Check sheet for the modelled part. Datum: model origin and axes. Units: mm. A direction names the side the tool comes from. Round coordinates to 2 decimals unless told otherwise and drop trailing zeros. Write each loop counter-clockwise with the first axis right and the second up, starting at its lowest first coordinate (ties: lowest second). Pieces come first, ordered by that corner, then holes. Notation, with made-up numbers: (37, -3) - (44, -3) arc R18 ccw to (44, 2) - close; hole circle Ø11 at (75, 64.5). An arc over 180 degrees is marked (long way). Answer as a JSON object with one key per item and string values. Group by question number.
Item 1: Sectioned sample at C-C on z = 1.5. Record the boundary of the cut face in (x, y), plus the area to 3 significant figures.
Item 2: Sectioned sample at B-B on x = 0. Record the boundary of the cut face in (y, z) (3 decimals), plus the area to 3 significant figures.
Item 3: Thickness scan on line 1 (Z direction, x = 0, y = 7.2); line 2 (X direction, y = 1.25, z = 1.25). Record the ranges inside material, lowest first.
Item 4: Sectioned sample at A-A on y = 4. Record the boundary of the cut face in (x, z).
Item 5: Release check for a two-part mould opening along X. For faces 3 (the flat face through (0, 3, -1)), 4 (the flat face through (0, 0, 0)) record: pulls with the +X half, pulls with the -X half, needs draft (parallel to the pull), parting line crosses it, or undercut.
Item 6: Gauge pin test, flat ends, axial feed: P1, Ø0.5, axis at x = -0.5, z = -1.5, coming from the -Y side; P2, Ø4, axis at x = 0, z = 0, coming from the -Y side; P3, Ø1.4, axis at x = -0.5, z = -0.5, coming from the +Y side; P4, Ø1, axis at x = -1, y = 4, coming from the +Z side. Record the tip position at first contact, or that the pin passes through.
Item 7: Set-up check for faces 1 (the flat face through (0, 1, -0.45)), 2 (the cylindrical face through (1.29, 6.595, -2.024)): record each of +Z, -Z, +X, -X, +Y, -Y from which the full face is reachable in a straight line by a thin tool's end or side.
Item 8: Sectioned sample at D-D on x = 2.25. Record the boundary of the cut face in (y, z).
Autodesk Inventor part; units mm, degrees
ref_plane "YZ Plane" through (0, 0, 0) normal (1, 0, 0) x (0, 1, 0)
ref_plane "XZ Plane" through (0, 0, 0) normal (0, 1, 0) x (-1, 0, 0)
ref_plane "XY Plane" through (0, 0, 0) normal (0, 0, 1) x (1, 0, 0)
sketch "Sketch1" plane through (0, 0, 0) normal (0, 1, 0) x (-1, 0, 0)
  circle A0 centre (0, 0) radius 1.975
  circle A1 centre (0, 0) radius 3.5
  line L0 (-2.286, -0.45) -> (2.286, -0.45)
  line L1 (2.286, -0.45) -> (2.286, 0.45)
  line L2 (2.286, 0.45) -> (-2.286, 0.45)
  line L3 (-2.286, 0.45) -> (-2.286, -0.45)
  line L4 (-2.286, -0.45) -> (2.286, 0.45) construction
  line L5 (2.286, -0.45) -> (-2.286, 0.45) construction
  point P0 (-1.9231, 0.45)
  point P1 (1.9231, 0.45)
  point P2 (1.9231, -0.45)
  point P3 (-1.9231, -0.45)
  dimension "d0" = 3.95
  dimension "d1" = 7
  dimension "d2" = 0.9
  dimension "d10" = 4.572
extrude "Extrusion1" add sketch "Sketch1" along normal blind 3 contours A0 L0 L2 | A0 L2 L1 L0 | A0 L0 L3 L2 | A1
sketch "Sketch2" plane through (0, 3, 0) normal (0, 1, 0) x (1, 0, 0)
  circle A0 centre (0, 0) radius 3.5
extrude "Extrusion2" add sketch "Sketch2" along normal blind 6.35
sketch "Sketch3" plane through (0, 9.35, 0) normal (0, 1, 0) x (1, 0, 0)
  circle A0 centre (0, 0) radius 2.4
  dimension "d7" = 4.8
extrude "Extrusion3" cut sketch "Sketch3" against normal blind 5.588
properties part number "TurnBot"
Completed:
{
 "1": {"outline": "(-3.16, 0) - (-1.28, 0) - (-1.28, 3) - (1.28, 3) - (1.28, 0) - (3.16, 0) - (3.16, 9.35) - (1.87, 9.35) - (1.87, 3.76) - (-1.87, 3.76) - (-1.87, 9.35) - (-3.16, 9.35) - close", "area": "30.5 mm²"},
 "2": {"outline": "(0, -3.5) - (9.35, -3.5) - (9.35, -2.4) - (3.762, -2.4) - (3.762, 2.4) - (9.35, 2.4) - (9.35, 3.5) - (0, 3.5) - (0, 1.975) - (3, 1.975) - (3, 0.45) - (0, 0.45) - (0, -0.45) - (3, -0.45) - (3, -1.975) - (0, -1.975) - close", "area": "29.5 mm²"},
 "3": {"line 1": "-3.5 to -2.4, 2.4 to 3.5", "line 2": "-3.27 to -1.53, 1.53 to 3.27"},
 "4": {"outline": "circle Ø7 at (0, 0); hole circle Ø4.8 at (0, 0)"},
 "5": {"face 3": "undercut", "face 4": "needs draft"},
 "6": {"P1": "y = 3", "P2": "y = 0", "P3": "y = 3.76", "P4": "z = 3.46"},
 "7": {"face 1": "-Y", "face 2": "+Y"},
 "8": {"outline": "(0, -2.68) - (9.35, -2.68) - (9.35, -0.84) - (3.76, -0.84) - (3.76, 0.84) - (9.35, 0.84) - (9.35, 2.68) - (0, 2.68) - close"}
}
